CAD build for the part. Positions are in the model's coordinates, mm. Coordinates: 2 decimals unless noted, no trailing zeros. Order: outer loops, then holes, each group sorted by start corner. A loop starts at its lowest first (then second) coordinate and runs counter-clockwise, first axis right, second up. Notation, with made-up numbers: (53.5, -4) - (84.5, -4) arc R9 ccw to (84.5, 10) - close; hole circle Ø11 at (-39, -30). An arc over 180 degrees is marked (long way). Return JSON: item names as keys, results as strings.
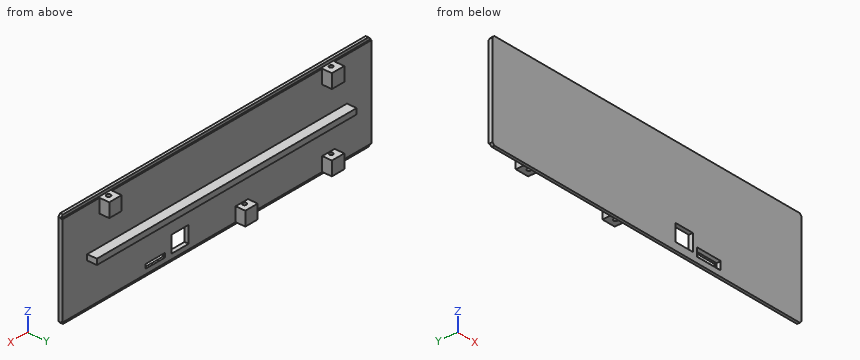
from build123d import *

# Parameters (mm, degrees)
SKETCH006_W     = 250
SKETCH006_H     = 65
PAD003_DEPTH    = 3
SKETCH014_W     = 14
SKETCH014_H     = 12
SKETCH014_W_2   = 16
SKETCH014_H_2   = 3
POCKET006_DEPTH = 5
SKETCH029_W     = 10
SKETCH029_H     = 8
PAD010_DEPTH    = 10
SKETCH034_W     = 10
SKETCH034_H     = 8
PAD012_DEPTH    = 10
SKETCH038_R     = 1.496657
SKETCH038_R_2   = 1.36472
POCKET040_DEPTH = 11
SKETCH030_R     = 1.4
POCKET041_DEPTH = 14
SKETCH041_W     = 210
SKETCH041_H     = 4
PAD022_DEPTH    = 7
SKETCH042_W     = 2
SKETCH042_H     = 2
PAD023_DEPTH    = 250
CHAMFER036_SIZE = 1.5


with BuildPart() as part:
    # Sketch006 → Pad003 (new body)
    with BuildSketch(Plane.XZ):
        Rectangle(SKETCH006_W, SKETCH006_H)
    extrude(amount=PAD003_DEPTH)

    # Sketch014 (on Face6 of Pad003) → Pocket006 (cut)
    with BuildSketch(Plane.XZ.offset(3)):
        with Locations((30, -23)):
            Rectangle(SKETCH014_W, SKETCH014_H)
        with Locations((50, -27.5)):
            Rectangle(SKETCH014_W_2, SKETCH014_H_2)
    extrude(amount=-POCKET006_DEPTH, mode=Mode.SUBTRACT)

    # Sketch029 (on Face1 of Pocket006) → Pad010 (join)
    with BuildSketch(Plane(origin=(0, 0, 32.5), x_dir=(-1, 0, 0), z_dir=(0, 0, 1))):
        with Locations((-90, -3)):
            Rectangle(SKETCH029_W, SKETCH029_H)
        with Locations((90, -3)):
            Rectangle(SKETCH029_W, SKETCH029_H)
    extrude(amount=-PAD010_DEPTH)

    # Sketch034 → Pad012 (join)
    with BuildSketch(Plane(origin=(0, 0, -32.5), x_dir=(1, 0, 0), z_dir=(0, 0, -1))):
        with Locations((-20, -3)):
            Rectangle(SKETCH034_W, SKETCH034_H)
        with Locations((-90, -3)):
            Rectangle(SKETCH034_W, SKETCH034_H)
    extrude(amount=-PAD012_DEPTH)

    # Sketch038 (on Face30 of Pad012) → Pocket040 (cut)
    with BuildSketch(Plane(origin=(0, 0, 32.5), x_dir=(-1, 0, 0), z_dir=(0, 0, 1))):
        with Locations((-90, -2)):
            Circle(SKETCH038_R)
        with Locations((90, -2)):
            Circle(SKETCH038_R_2)
    extrude(amount=-POCKET040_DEPTH, mode=Mode.SUBTRACT)

    # Sketch030 → Pocket041 (cut)
    with BuildSketch(Plane(origin=(0, 0, -32.5), x_dir=(1, 0, 0), z_dir=(0, 0, -1))):
        with Locations((-20, -2)):
            Circle(SKETCH030_R)
        with Locations((-90, -2)):
            Circle(SKETCH030_R)
    extrude(amount=-POCKET041_DEPTH, mode=Mode.SUBTRACT)

    # Sketch041 → Pad022 (join)
    with BuildSketch(Plane(origin=(0, 0, 0), x_dir=(1, 0, 0), z_dir=(0, 1, 0))):
        with Locations((0, 0.5)):
            Rectangle(SKETCH041_W, SKETCH041_H)
    extrude(amount=PAD022_DEPTH)

    # Sketch042 → Pad023 (join)
    with BuildSketch(Plane(origin=(-125, 0, 0), x_dir=(0, 0, -1), z_dir=(-1, 0, 0))):
        with Locations((33.5, 2)):
            Rectangle(SKETCH042_W, SKETCH042_H)
    pad023 = extrude(amount=-PAD023_DEPTH)

    # Mirrored007: Pad023 across Sketch042 V_Axis
    add(pad023.mirror(Plane(origin=(-125, 0, 0), x_dir=(-1, 0, 0), z_dir=(0, 0, -1))))

    # Chamfer036
    chamfer036_edges = [part.edges().sort_by_distance(p)[0] for p in [
        (50, -3, -26),
        (58, -3, -27.5),
        (42, -3, -27.5),
        (50, -3, -29),
        (125, -2, -34.5),
        (125, -2, 34.5),
        (-125, -2, 34.5),
        (-125, -2, -34.5),
    ]]
    chamfer(chamfer036_edges, length=CHAMFER036_SIZE)


with BuildPart() as part_1:
    # Body002 placement: moved
    add(part.part.moved(Location((0, -77, 0))))


solid = part_1.part
Item 1: Drop flat-ended pins along their axis: P1, Ø6, axis at y = -76.5, z = -7, coming from the +X side; P2, Ø1.5, axis at x = -13, z = 11, coming from the +Y side; P3, Ø2, axis at x = -90, y = -75, coming from the -Z side; P4, Ø3.5, axis at x = -21.5, y = -74, coming from the +Z side. Give the stop position or say it passes through.
Findings below:
{"P1": "stops at x = 125", "P2": "stops at y = -77", "P3": "stops at z = -2.5", "P4": "stops at z = 1.5"}
Item 2: Band-saw the part on D-D, the plane x = 55. List the corners of the cut face in (y, z).
Findings below:
{"outline": "(-80, -34.5) - (-78, -34.5) - (-78, -32.5) - (-77, -32.5) - (-77, -29) - (-78.5, -29) - (-80, -30.5) - close; (-80, -24.5) - (-78.5, -26) - (-77, -26) - (-77, -2.5) - (-70, -2.5) - (-70, 1.5) - (-77, 1.5) - (-77, 32.5) - (-78, 32.5) - (-78, 34.5) - (-80, 34.5) - close"}
Item 3: Wall check: L1, parallel to X at y = -75, z = -27; L2, parallel to Y at x = 90, z = 30; L3, parallel to Z at x = 91.5, y = -71.75. Give the ranges that are in metal, low to high. Write a range as [from, to].
Findings below:
{"L1": "x = [-95, -91.4], [-88.6, -85], [-25, -21.4], [-18.6, -15]", "L2": "y = [-80, -76.5], [-73.5, -70]", "L3": "z = [-2.5, 1.5], [22.5, 32.5]"}
Item 4: Band-saw the part on B-B, the plane y = -72. List the corners of the cut face in (x, z), then the cut area to 3 significant figures.
Findings below:
{"outline": "(-105, -2.5) - (105, -2.5) - (105, 1.5) - (-105, 1.5) - close; (-95, -32.5) - (-85, -32.5) - (-85, -22.5) - (-95, -22.5) - close; (-95, 22.5) - (-85, 22.5) - (-85, 32.5) - (-95, 32.5) - close; (-25, -32.5) - (-15, -32.5) - (-15, -22.5) - (-25, -22.5) - close; (85, 22.5) - (95, 22.5) - (95, 32.5) - (85, 32.5) - close", "area": "1,240 mm²"}
Item 5: Band-saw the part on C-C, the plane x = -98. List the corners of the cut face in (y, z).
Findings below:
{"outline": "(-80, -34.5) - (-78, -34.5) - (-78, -32.5) - (-77, -32.5) - (-77, -2.5) - (-70, -2.5) - (-70, 1.5) - (-77, 1.5) - (-77, 32.5) - (-78, 32.5) - (-78, 34.5) - (-80, 34.5) - close"}
Item 6: Band-saw the part on A-A, the plane x = 29. List the corners of the cut face in (y, z), then the cut area to 3 significant figures.
Findings below:
{"outline": "(-80, -34.5) - (-78, -34.5) - (-78, -32.5) - (-77, -32.5) - (-77, -29) - (-80, -29) - close; (-80, -17) - (-77, -17) - (-77, -2.5) - (-70, -2.5) - (-70, 1.5) - (-77, 1.5) - (-77, 32.5) - (-78, 32.5) - (-78, 34.5) - (-80, 34.5) - close", "area": "195 mm²"}
